from build123d import *

# Parameters (mm, degrees)
SKETCH1_R           = 6.5484375
SKETCH1_R_2         = 4.9609375
BOSS_EXTRUDE1_DEPTH = 15.875
CUT_EXTRUDE1_DEPTH  = 3.175


with BuildPart() as part:
    # Sketch1 → Boss-Extrude1 (new body)
    with BuildSketch(Plane.XY):
        with BuildLine():
            Line((39.309837535, -38.13576648), (169.802643178, 71.308446723))
            ThreePointArc((169.802643178, 71.308446723), (181.638701023, 75.538599133), (193.375235205, 71.039685917))
            ThreePointArc((193.375235205, 71.039685917), (194.91888163, 70.411561678), (196.519579076, 70.875406513))
            ThreePointArc((196.519579076, 70.875406513), (216.426062494, 95.878722868), (219.876867623, 127.651759468))
            ThreePointArc((219.876867623, 127.651759468), (216.10638338, 133.218163447), (209.442132072, 134.106509769))
            Line((209.442132072, 134.106509769), (169.802643178, 97.116806131))
            ThreePointArc((169.802643178, 97.116806131), (141.448926781, 73.105263596), (110.917160699, 51.932198905))
            Line((110.917160699, 51.932198905), (61.60231529, 21.139969158))
            ThreePointArc((61.60231529, 21.139969158), (33.929413541, 11.389122801), (4.735454932, 14.318504397))
            ThreePointArc((4.735454932, 14.318504397), (-13.47453995, 6.773542256), (-8.666712343, -12.34229309))
            Line((-8.666712343, -12.34229309), (28.215623228, -38.240932071))
            ThreePointArc((28.215623228, -38.240932071), (33.77962274, -39.970371676), (39.309837535, -38.13576648))
        make_face()
        Circle(SKETCH1_R, mode=Mode.SUBTRACT)
        with Locations((38.1, -5.431682667)):
            Circle(SKETCH1_R_2, mode=Mode.SUBTRACT)
    extrude(amount=BOSS_EXTRUDE1_DEPTH)

    # Sketch2 → Cut-Extrude1 (cut)
    with BuildSketch(Plane(origin=(0, 0, 0), x_dir=(-1, 0, 0), z_dir=(0, 0, -1))):
        with BuildLine():
            Line((-174.134916332, 92.474187331), (-212.247088608, 128.038671053))
            ThreePointArc((-212.247088608, 128.038671053), (-213.153727633, 127.498423524), (-213.622663407, 126.552928441))
            ThreePointArc((-213.622663407, 126.552928441), (-211.065734224, 99.589440169), (-195.076715953, 77.728084278))
            ThreePointArc((-195.076715953, 77.728084278), (-180.13970514, 81.855576515), (-165.722085208, 76.173788093))
            Line((-165.722085208, 76.173788093), (-67.427567629, -6.265746298))
            ThreePointArc((-67.427567629, -6.265746298), (-58.337399342, -8.416558755), (-51.185588969, -2.40750208))
            ThreePointArc((-51.185588969, -2.40750208), (-51.037402279, 5.455937622), (-56.434934077, 11.176277972))
            ThreePointArc((-56.434934077, 11.176277972), (-60.775393958, 13.324892332), (-64.965487459, 15.753729935))
            Line((-64.965487459, 15.753729935), (-114.280332868, 46.545959683))
            ThreePointArc((-114.280332868, 46.545959683), (-145.314571941, 68.067477625), (-174.134916332, 92.474187331))
        make_face()
    cut_extrude1 = extrude(amount=-CUT_EXTRUDE1_DEPTH, mode=Mode.SUBTRACT)

    # Mirror1: Cut-Extrude1 across plane
    add(cut_extrude1.mirror(Plane(origin=(0, 0, 7.9375), x_dir=(1, 0, 0), z_dir=(0, 0, -1))), mode=Mode.SUBTRACT)


solid = part.part
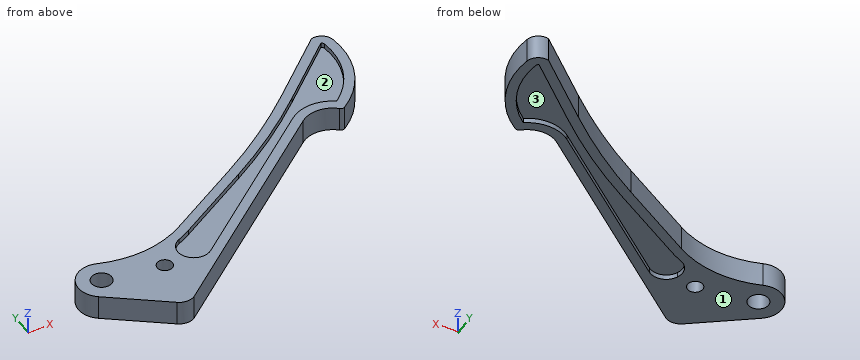
Design review of the part built by this model. Coordinates are the model's own, in mm. Face numbers are marked on the shaded views. A direction names the side the tool comes from. Give positions to 0.01 mm unless a question says otherwise; leave off trailing zeros. Write each loop counter-clockwise with the first axis right and the second up, starting at its lowest first coordinate (ties: lowest second). Pieces come first, ordered by that corner, then holes. Notation, with made-up numbers: M -8.5,-38.5 L 8.5,-38.5 A12 ccw 8.5,-26.5 Z; hole C 69.5,27.25 d1. An arc over 180 degrees is marked long. Return JSON: item names as keys, results as strings. Group by question number.
Item 1: Tool access review of the marked faces 1, 2 and 3: name each direction out of +Z, -Z, +X, -X, +Y, -Y from which nothing blocks a thin tool from reaching the whole face with its end or side.
Item 2: Wall thickness on line 1 along X through (y, z) = (104.5, 1.5); line 2 along Y through (x, z) = (38.1, 5.5); line 3 along Z through (x, y) = (181.5, 88.5) (3 decimals): over which ranges is each line inside the solid? List them lowest first.
Item 3: Take a section at B-B (x = 0). Give the boundary of the cut face in (y, z) (3 decimals), plus the area to 3 significant figures.
Item 4: Take a section at C-C (y = 35.5). Give the boundary of the cut face in (x, z) (3 decimals).
Item 5: Take a section at D-D (x = 204). Give the boundary of the cut face in (y, z) (3 decimals), plus the area to 3 significant figures.
Item 6: Take a section at A-A (z = 7.5). Count the separate pieces of the cut face and the enclosed holes in it, plus the area to 3 significant figures.
Item 7: Clearance check with flat-ended pins moving along their axes: pin 1 Ø8 at (x, z) = (55.5, 7.5) entering from +Y; pin 2 Ø6 at (x, z) = (153.5, 12) entering from +Y; pin 3 Ø8 at (x, y) = (64.5, 2.5) entering from +Z. State where each tip first meets the part, or that it passes through.
Return value:
{
 "1": {"face 1": "-Z, +X, -X, +Y, -Y", "face 2": "+Z", "face 3": "-Z"},
 "2": {"line 1": "x = 177.71 to 187.02, 212.65 to 219.2", "line 2": "y = -38.89 to -10.39, -0.47 to 12.02", "line 3": "z = 3.175 to 12.7"},
 "3": {"outline": "M -18.428,0 L -6.548,0 L -6.548,15.875 L -18.428,15.875 Z; M 6.548,0 L 15.081,0 L 15.081,15.875 L 6.548,15.875 Z", "area": "324 mm2"},
 "4": {"outline": "M 84.6,0 L 96.59,0 L 96.59,3.175 L 117.226,3.175 L 117.226,0 L 127.107,0 L 127.107,15.875 L 117.226,15.875 L 117.226,12.7 L 96.59,12.7 L 96.59,15.875 L 84.6,15.875 Z"},
 "5": {"outline": "M 77.198,0 L 86.845,0 L 86.845,3.175 L 120.343,3.175 L 120.343,0 L 129.028,0 L 129.028,15.875 L 120.343,15.875 L 120.343,12.7 L 86.845,12.7 L 86.845,15.875 L 77.198,15.875 Z", "area": "610 mm2"},
 "6": {"separate pieces": "1", "enclosed holes": "2", "area": "8,210 mm2"},
 "7": {"pin 1": "stops at y = 19.88", "pin 2": "stops at y = 85.27", "pin 3": "stops at z = 12.7"}
}
